```python
from build123d import *

# Parameters (mm, degrees)
BOSS_EXTRUDE1_DEPTH     = 4.445
CUT_EXTRUDE1_REACH      = 13.535
CUT_EXTRUDE1_END_RADIUS = 41.91
SKETCH2_W               = 9.8425
SKETCH2_H               = 8.255
CUT_EXTRUDE3_REACH      = 14.779
CUT_EXTRUDE3_END_RADIUS = 43.18
SKETCH3_W               = 9.525
SKETCH3_H               = 8.255
BOSS_EXTRUDE2_REACH     = 15.825
SKETCH4_R               = 2.54
SKETCH4_R_2             = 1.905
SKETCH5_W               = 6.203096786
SKETCH5_H               = 3.175
CUT_EXTRUDE4_DEPTH      = 13.197951714
CUT_EXTRUDE4_DEPTH_BACK = 13.197951714


with BuildPart() as part:
    # Sketch1 → Boss-Extrude1 (new, symmetric)
    with BuildSketch(Plane.XY):
        with BuildLine():
            Line((-10.16, 0), (-10.16, 3.175))
            ThreePointArc((-10.16, 3.175), (0.312688289, 1.885753156), (10.16, -1.905))
            Line((10.16, -1.905), (10.16, -3.175))
            Line((10.16, -3.175), (0, -3.175))
            Line((0, -3.175), (0, 0))
            Line((0, 0), (-10.16, 0))
        make_face()
    extrude(amount=BOSS_EXTRUDE1_DEPTH, both=True)

    # Cut-Extrude1: up to this cylinder (the profile starts inside it)
    cut_extrude1_end = Plane(origin=(-10.16, -40.005, 0), z_dir=(0, 0, -1)) * Cylinder(CUT_EXTRUDE1_END_RADIUS, 111.89, mode=Mode.PRIVATE)
    # Sketch2 → Cut-Extrude1 (cut, up to the surface)
    with BuildSketch(Plane.XZ, mode=Mode.PRIVATE) as cut_extrude1_sk1:
        with Locations((-4.92125, 0)):
            Rectangle(SKETCH2_W, SKETCH2_H)
    cut_extrude1_tool1 = extrude(cut_extrude1_sk1.sketch, amount=-CUT_EXTRUDE1_REACH, mode=Mode.PRIVATE) & cut_extrude1_end
    add(cut_extrude1_tool1.solids().sort_by_distance((-4.92125, 0, 0))[0], mode=Mode.SUBTRACT)

    # Cut-Extrude3: up to this cylinder (the profile starts inside it)
    cut_extrude3_end = Plane(origin=(-10.16, -41.275, 0), z_dir=(0, 0, -1)) * Cylinder(CUT_EXTRUDE3_END_RADIUS, 116.918, mode=Mode.PRIVATE)
    # Sketch3 → Cut-Extrude3 (cut, up to the surface)
    with BuildSketch(Plane.XZ.offset(3.175), mode=Mode.PRIVATE) as cut_extrude3_sk1:
        with Locations((5.08, 0)):
            Rectangle(SKETCH3_W, SKETCH3_H)
    cut_extrude3_tool1 = extrude(cut_extrude3_sk1.sketch, amount=-CUT_EXTRUDE3_REACH, mode=Mode.PRIVATE) & cut_extrude3_end
    add(cut_extrude3_tool1.solids().sort_by_distance((5.08, -3.175, 0))[0], mode=Mode.SUBTRACT)

    # Sketch4 → Boss-Extrude2 (add, up to next)
    with BuildSketch(Plane(origin=(0, -5.08, 0), x_dir=(1, 0, 0), z_dir=(0, 1, 0)), mode=Mode.PRIVATE) as boss_extrude2_sk1:
        with Locations(Location((-5.08, 0, 0), (0, 0, 90))):
            Circle(SKETCH4_R)
        with Locations(Location((-5.08, 0, 0), (0, 0, 90))):
            Circle(SKETCH4_R_2, mode=Mode.SUBTRACT)
    boss_extrude2_tool1 = extrude(boss_extrude2_sk1.sketch, amount=BOSS_EXTRUDE2_REACH, mode=Mode.PRIVATE) - part.part
    # Sketch4 → Boss-Extrude2 (add, up to next)
    with BuildSketch(Plane(origin=(0, -5.08, 0), x_dir=(1, 0, 0), z_dir=(0, 1, 0)), mode=Mode.PRIVATE) as boss_extrude2_sk2:
        with Locations(Location((5.08, 0, 0), (0, 0, 90))):
            Circle(SKETCH4_R)
        with Locations(Location((5.08, 0, 0), (0, 0, 90))):
            Circle(SKETCH4_R_2, mode=Mode.SUBTRACT)
    boss_extrude2_tool2 = extrude(boss_extrude2_sk2.sketch, amount=BOSS_EXTRUDE2_REACH, mode=Mode.PRIVATE) - part.part
    add(boss_extrude2_tool1.solids().sort_by_distance((-5.08, -5.08, 2.468158))[0])
    add(boss_extrude2_tool2.solids().sort_by_distance((5.08, -5.08, 2.468158))[0])

    # Sketch5 → Cut-Extrude4 (cut, two sides)
    with BuildSketch(Plane.XY) as cut_extrude4_sk:
        with Locations((-4.842768544, -3.4925)):
            Rectangle(SKETCH5_W, SKETCH5_H)
    extrude(amount=CUT_EXTRUDE4_DEPTH, mode=Mode.SUBTRACT)
    extrude(cut_extrude4_sk.sketch, amount=-CUT_EXTRUDE4_DEPTH_BACK, mode=Mode.SUBTRACT)


solid = part.part
```
Can you work these out from the model? Positions are in its coordinate system, mm. A direction names the side the tool comes from. Give positions to 0.01 mm unless a question says otherwise; leave off trailing zeros. Order: outer loops, then holes, each group sorted by start corner. A loop starts at its lowest first (then second) coordinate and runs counter-clockwise, first axis right, second up. Notation, with made-up numbers: M -29,37.25 L -12,37.25 A29 ccw -12,61.25 Z; hole C 58,39 d6. An arc over 180 degrees is marked long. Write item = value, one per line. Start each with the question number.
Q1. I need wall thicknesses on probe 1 along Z at (x, y) = (2, -1.25) (1 decimal); probe 2 along X at (y, z) = (-2, -0.75); probe 3 along X at (y, z) = (-2.5, 1.25). Which ranges of each line are inside material? Lowest first, please. Write a range as [from, to].
Q2. Will these pins go through, and if not, where does the flat tip stop? pin 1 Ø4 at (x, z) = (-6.5, -0.5) entering from +Y; pin 2 Ø1.5 at (x, z) = (-6.5, 2) entering from -Y (3 decimals); pin 3 Ø2.5 at (x, z) = (-5.08, 0) entering from +Y.
Q3. We'd pull the mould along X, two halves only. Please class faces 5 (the cylindrical face through (5.07, -0.87, -0.03)), 6 (the cylindrical face through (0.17, 1.92, 0.06)), 7 (the flat face through (0, 1, -4.445)): pulls with the +X half, pulls with the -X half, needs draft (parallel to the pull), parting line crosses it, or undercut.
Q4. Suppose I cut it at A-A (y = -1.25). Write out the boundary of the cut face in (x, z) (1 decimal), plus the area to 3 significant figures.
Q5. For faces 1 (the cylindrical face through (-6.97, -0.09, 0.25)), 2 (the flat face through (-4, -1.905, 2)), 3 (the flat face through (0, 1, 4.445)), 4 (the flat face through (-10, 0, 0)), which set-ups out of +Z, -Z, +X, -X, +Y, -Y let a thin tool reach every point of the face, with its end or its side?
Check result:
q1.probe_1 = [-4.4, -4.1], [4.1, 4.4]
q1.probe_2 = [0, 0.32], [2.65, 3.33], [6.83, 7.51], [7.78, 10.16]
q1.probe_3 = [0, 0.32], [2.87, 3.64], [6.52, 7.29], [8.84, 10.16]
q2.pin_1 = 3.14
q2.pin_2 = -1.905
q2.pin_3 = 3
q3.face_5 = undercut
q3.face_6 = pulls with the +X half
q3.face_7 = needs draft
q4.outline = C -5.1,0 d5.1; M 0,-4.4 L 8.9,-4.4 L 8.9,4.4 L 0,4.4 Z; hole C -5.1,0 d3.8; hole M 0.3,-4.1 L 6,-4.1 L 6,-2.4 A2.5 cw long 6,2.4 L 6,4.1 L 0.3,4.1 Z; hole M 6,-1.6 L 6,1.6 A1.9 ccw long Z
q4.area = 46.3 mm2
q5.face_1 = -Y
q5.face_2 = +Z, -Z, -X, -Y
q5.face_3 = +Z, +X, -X, +Y, -Y
q5.face_4 = -X, -Y
